Input: part model. Units: mm. Frame: model coordinates. Face numbers are marked on the shaded views. Give positions to 0.01 mm unless a question says otherwise; leave off trailing zeros. Write each loop counter-clockwise with the first axis right and the second up, starting at its lowest first coordinate (ties: lowest second). Pieces come first, ordered by that corner, then holes.
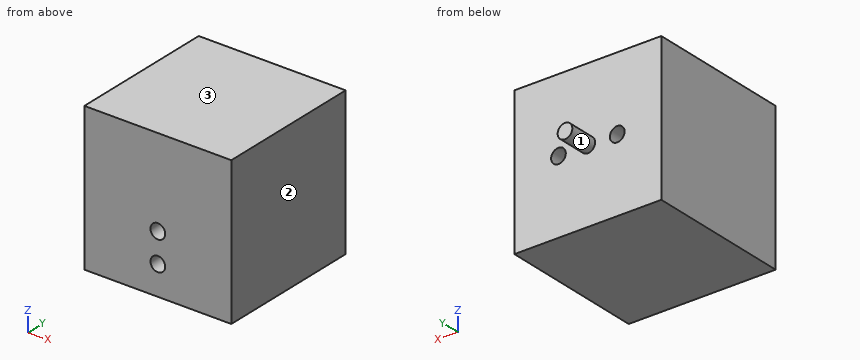
```python
from build123d import *

# Parameters (mm, degrees)
F0_W     = 63.5
F0_H     = 63.5
F1_DEPTH = 63.5
F2_R     = 3.175
F3_DEPTH = 12.7
F4_DEPTH = 12.7
F5_R     = 3.175
F6_DEPTH = 12.7


with BuildPart() as f1:
    # F0 (on Top) → F1 (new body)
    with BuildSketch(Plane.XY):
        Rectangle(F0_W, F0_H)
    extrude(amount=F1_DEPTH)

    # F2 (on face) → F3 (join)
    with BuildSketch(Plane(origin=(0, 31.75, 0), x_dir=(-1, 0, 0), z_dir=(0, 1, 0))):
        with Locations((0, 31.75)):
            Circle(F2_R)
    extrude(amount=F3_DEPTH)

    # F2 (on face) → F4 (cut)
    with BuildSketch(Plane(origin=(0, 31.75, 0), x_dir=(-1, 0, 0), z_dir=(0, 1, 0))):
        with Locations((-12.7, 31.75)):
            Circle(F2_R)
        with Locations((12.7, 31.75)):
            Circle(F2_R)
    extrude(amount=-F4_DEPTH, mode=Mode.SUBTRACT)

    # F5 (on face) → F6 (cut)
    with BuildSketch(Plane.XZ.offset(31.75)):
        with Locations((0, 25.4)):
            Circle(F5_R)
        with Locations((0, 12.7)):
            Circle(F5_R)
    extrude(amount=-F6_DEPTH, mode=Mode.SUBTRACT)


solid = f1.part
```
Item 1: Section A-A (y = 25). Return loops of the section in (x, z) (3 decimals).
Item 2: Section C-C (z = 31.75). Return loops of the section in (x, y) (3 decimals).
Item 3: Section D-D (z = 56). Return loops of the section in (x, y), and give its area (3 significant figures).
Item 4: Mould query, pull axis Z, two halves, no side actions, for the marked faces 1, 2 and 3. Classes: +Z half, -Z half, draft (parallel to the pull), parting line (faces both ways), or undercut.
Item 5: Ray query, line 1 (Z direction, x = 0, y = -25.25) (3 decimals); line 2 (X direction, y = 28, z = 31); line 3 (Z direction, x = 12.7, y = 25.25) (3 decimals). Return the intervals inside material, ascending.
Item 6: Pin query (flat end, axial travel): pin 1 (8.5 mm diameter, centred on x = 0, z = 12.7, fed in from +Y); pin 2 (3 mm diameter, centred on x = 17, y = 20, fed in from -Z); pin 3 (1.9 mm diameter, centred on x = 1.5, z = 24, fed in from -Y). Return the tip coordinate at first contact, or that it passes through.
Item 7: Section B-B (x = 0). Return loops of the section in (y, z) (3 decimals), and give its area (3 significant figures).
Solved:
1. outline: (-31.75, 0) - (31.75, 0) - (31.75, 63.5) - (-31.75, 63.5) - close; hole circle Ø6.35 at (-12.7, 31.75); hole circle Ø6.35 at (12.7, 31.75)
2. outline: (-31.75, -31.75) - (31.75, -31.75) - (31.75, 31.75) - (15.875, 31.75) - (15.875, 19.05) - (9.525, 19.05) - (9.525, 31.75) - (3.175, 31.75) - (3.175, 44.45) - (-3.175, 44.45) - (-3.175, 31.75) - (-9.525, 31.75) - (-9.525, 19.05) - (-15.875, 19.05) - (-15.875, 31.75) - (-31.75, 31.75) - close
3. outline: (-31.75, -31.75) - (31.75, -31.75) - (31.75, 31.75) - (-31.75, 31.75) - close
3. area: 4,030 mm2
4. face 1: parting line
4. face 2: draft
4. face 3: +Z half
5. line 1: z = 0 to 9.525, 15.875 to 22.225, 28.575 to 63.5
5. line 2: x = -31.75 to -15.79, -9.61 to 9.61, 15.79 to 31.75
5. line 3: z = 0 to 28.575, 34.925 to 63.5
6. pin 1: stops at y = 31.75
6. pin 2: stops at z = 0
6. pin 3: stops at y = -19.05
7. outline: (-31.75, 0) - (31.75, 0) - (31.75, 28.575) - (44.45, 28.575) - (44.45, 34.925) - (31.75, 34.925) - (31.75, 63.5) - (-31.75, 63.5) - (-31.75, 28.575) - (-19.05, 28.575) - (-19.05, 22.225) - (-31.75, 22.225) - (-31.75, 15.875) - (-19.05, 15.875) - (-19.05, 9.525) - (-31.75, 9.525) - close
7. area: 3,950 mm2
